Work out the finished part from the listing and answer in its coordinate system (mm). Face numbers are marked on the shaded views. A direction names the side the tool comes from. Round coordinates to 2 decimals unless told otherwise and drop trailing zeros. Loops run counter-clockwise (first coordinate to the right, second up) from the corner with the lowest first, then second, coordinate; pieces in that order, holes last. Notation, with made-up numbers: (-16.75, 63) - (1.25, 63) arc R21 ccw to (1.25, 90) - close; hole circle Ø8 at (55.5, 71). An arc over 180 degrees is marked (long way). Use CSV: the item, a comma, the result in double quotes. Start each with the question number.
from build123d import *

# Parameters (mm, degrees)
SKETCH1_W           = 75
SKETCH1_H           = 43
SKETCH1_R           = 1.5
BOSS_EXTRUDE1_DEPTH = 1.5
SKETCH3_W           = 5.662945026
SKETCH3_H           = 23.11722764
BOSS_EXTRUDE2_DEPTH = 10
SKETCH4_W           = 2.260398275
SKETCH4_H           = 2.806011651
BOSS_EXTRUDE3_DEPTH = 5
SKETCH5_R           = 3.292125191
BOSS_EXTRUDE4_DEPTH = 15


with BuildPart() as part:
    # Sketch1 → Boss-Extrude1 (new body)
    with BuildSketch(Plane(origin=(0, 0, 0), x_dir=(1, 0, 0), z_dir=(0, 1, 0))):
        Rectangle(SKETCH1_W, SKETCH1_H)
        with Locations((-34.5, 17.5)):
            Circle(SKETCH1_R, mode=Mode.SUBTRACT)
        with Locations((-34.5, -17.5)):
            Circle(SKETCH1_R, mode=Mode.SUBTRACT)
        with Locations((34.5, -17.5)):
            Circle(SKETCH1_R, mode=Mode.SUBTRACT)
        with Locations((34.5, 17.5)):
            Circle(SKETCH1_R, mode=Mode.SUBTRACT)
    extrude(amount=BOSS_EXTRUDE1_DEPTH)

    # Sketch3 → Boss-Extrude2 (add)
    with BuildSketch(Plane(origin=(0, 1.5, 0), x_dir=(1, 0, 0), z_dir=(0, 1, 0))):
        with Locations((-33.163136966, 1.163618841)):
            Rectangle(SKETCH3_W, SKETCH3_H)
    extrude(amount=BOSS_EXTRUDE2_DEPTH)

    # Sketch4 → Boss-Extrude3 (add)
    with BuildSketch(Plane(origin=(0, 1.5, 0), x_dir=(1, 0, 0), z_dir=(0, 1, 0))):
        with Locations((34.903340681, 7.794476809)):
            Rectangle(SKETCH4_W, SKETCH4_H)
    extrude(amount=BOSS_EXTRUDE3_DEPTH)

    # Sketch5 → Boss-Extrude4 (add)
    with BuildSketch(Plane(origin=(0, 1.5, 0), x_dir=(1, 0, 0), z_dir=(0, 1, 0))):
        with Locations((-23.505100586, 16.988835077)):
            Circle(SKETCH5_R)
    extrude(amount=BOSS_EXTRUDE4_DEPTH)


solid = part.part
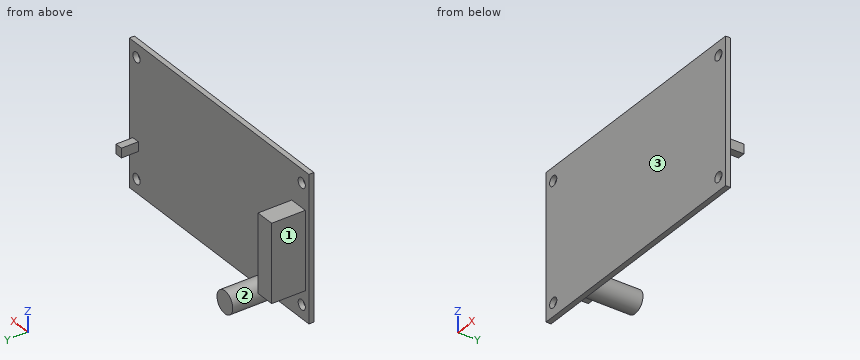
Item 1: Find the intervals of material crossed by probe 1 along Z at (x, y) = (-34.5, 0.35); probe 2 along X at (y, z) = (0.3, 17.5); probe 3 along Y at (x, z) = (21.5, -9), in increasing order. Write a range as [from, to].
Item 2: Each of these flat-tipped pins is pushed along its axis until it touches: pin 1 Ø2 at (y, z) = (5, -8) entering from -X; pin 2 Ø1.1 at (x, y) = (34.5, 3.5) entering from +Z; pin 3 Ø1.5 at (x, y) = (-27, 13.5) entering from +Z; pin 4 Ø1.5 at (x, y) = (-19, 5) entering from +Z. Where does it stop, or does it pass through?
Item 3: Which of the six approach directions +Z, -Z, +X, -X, +Y, -Y give full straight-line access (tool end or side, diameter ignored) to the marked faces 1, 2 and 3?
Item 4: A cutting plane is placed at C-C (y = 3.5). Determine the outline of the cut face in (x, z) (3 decimals), plus the area to 3 significant figures.
Item 5: A cutting plane is placed at B-B (z = 17.5). Determine the outline of the cut face in (x, y).
Item 6: A cutting plane is placed at A-A (x = 34.5). Determine the outline of the cut face in (y, z), plus the area to 3 significant figures.
Item 7: A cutting plane is placed at D-D (x = -34.5). Determine the outline of the cut face in (y, z) (3 decimals).
Result sheet:
1,probe 1,"[-21.5, -19], [-16, 16], [19, 21.5]"
1,probe 2,"[-37.5, -36], [-33, 33], [36, 37.5]"
1,probe 3,"[0, 1.5]"
2,pin 1,"x = -35.99"
2,pin 2,"z = -6.39"
2,pin 3,"z = -15.17"
2,pin 4,"through"
3,face 1,"+Z, -Z, -X, +Y"
3,face 2,"+Y"
3,face 3,"+Z, -Z, +X, -X, -Y"
4,outline,"(-35.995, -12.722) - (-30.332, -12.722) - (-30.332, 10.395) - (-35.995, 10.395) - close; circle Ø6.584 at (-23.505, -16.989); (33.773, -9.197) - (36.034, -9.197) - (36.034, -6.391) - (33.773, -6.391) - close"
4,area,"171 mm^2"
5,outline,"(-37.5, 0) - (-36, 0) - (-36, 1.5) - (-37.5, 1.5) - close; (-33, 0) - (33, 0) - (33, 1.5) - (-33, 1.5) - close; (36, 0) - (37.5, 0) - (37.5, 1.5) - (36, 1.5) - close"
6,outline,"(0, -21.5) - (1.5, -21.5) - (1.5, -19) - (0, -19) - close; (0, -16) - (1.5, -16) - (1.5, -9.2) - (6.5, -9.2) - (6.5, -6.39) - (1.5, -6.39) - (1.5, 16) - (0, 16) - close; (0, 19) - (1.5, 19) - (1.5, 21.5) - (0, 21.5) - close"
6,area,"69.5 mm^2"
7,outline,"(0, -21.5) - (1.5, -21.5) - (1.5, -19) - (0, -19) - close; (0, -16) - (1.5, -16) - (1.5, -12.722) - (11.5, -12.722) - (11.5, 10.395) - (1.5, 10.395) - (1.5, 16) - (0, 16) - close; (0, 19) - (1.5, 19) - (1.5, 21.5) - (0, 21.5) - close"
